from build123d import *

# Parameters (mm, degrees)
F0_W      = 20.75
F0_H      = 40.5
F2_DEPTH  = 2
F3_START  = 18
F1_W      = 20.75
F1_H      = 33.25
F3_DEPTH  = 2.25
F4_START  = -18
F4_DEPTH  = 2.25
F6_DEPTH  = 2.25
F8_DEPTH  = 2.25
F9_R      = 1.125
F10_DEPTH = 40.501
F11_R     = 1.27
F12_DEPTH = 2


with BuildPart() as f2:
    # F0 (on Top) → F2 (new body)
    with BuildSketch(Plane.XY):
        Rectangle(F0_W, F0_H)
    extrude(amount=F2_DEPTH)

    # F1 (on Front) → F3 (join)
    with BuildSketch(Plane.XZ.offset(F3_START)):
        with Locations((0, -16.625)):
            Rectangle(F1_W, F1_H)
    extrude(amount=F3_DEPTH)

    # F1 (on Front) → F4 (join)
    with BuildSketch(Plane.XZ.offset(F4_START)):
        with Locations((0, -16.625)):
            Rectangle(F1_W, F1_H)
    extrude(amount=-F4_DEPTH)

    # F5 (on face) → F6 (join, through all)
    with BuildSketch(Plane(origin=(0, 20.25, 0), x_dir=(-1, 0, 0), z_dir=(0, 1, 0))):
        Polygon((-10.375, -33.25), (-20.25, -33.25), (-20.25, -43.25), (20.25, -43.25), (20.25, -33.25), (10.375, -33.25), align=None)
    extrude(amount=-F6_DEPTH)

    # F7 (on face) → F8 (join, through all)
    with BuildSketch(Plane.XZ.offset(20.25)):
        Polygon((0, -33.25), (-20.25, -33.25), (-20.25, -43.25), (20.25, -43.25), (20.25, -33.25), align=None)
    extrude(amount=-F8_DEPTH)

    # F9 (on face) → F10 (cut, through all)
    with BuildSketch(Plane.XZ.offset(20.25)):
        with Locations((-13.25, -38.25)):
            Circle(F9_R)
        with Locations((13.25, -38.25)):
            Circle(F9_R)
    extrude(amount=-F10_DEPTH, mode=Mode.SUBTRACT)

    # F11 (on face) → F12 (cut, through all)
    with BuildSketch(Plane.XY.offset(2)):
        with BuildLine():
            ThreePointArc((-3.0697393815, 2.5959719896), (-3.3217599094, -8.4476517557), (6.286518813, -2.9973196771))
            ThreePointArc((6.286518813, -2.9973196771), (5.3868508916, 0.2609590453), (2.9427770074, 2.5959719896))
            ThreePointArc((2.9427770074, 2.5959719896), (-0.063481187, 0.0506803229), (-3.0697393815, 2.5959719896))
        make_face()
        with BuildLine():
            ThreePointArc((-3.0697393815, 2.5959719896), (-0.063481187, 3.3526803229), (2.9427770074, 2.5959719896))
            ThreePointArc((2.9427770074, 2.5959719896), (2.9740654362, 2.846461149), (2.984518813, 3.0986803229))
            ThreePointArc((2.984518813, 3.0986803229), (-0.315700361, 6.1362269461), (-3.0697393815, 2.5959719896))
        make_face()
        with BuildLine():
            ThreePointArc((-3.0697393815, 2.5959719896), (-0.063481187, 0.0506803229), (2.9427770074, 2.5959719896))
            ThreePointArc((2.9427770074, 2.5959719896), (-0.063481187, 3.3526803229), (-3.0697393815, 2.5959719896))
        make_face()
        with Locations((-0.063481187, -12.1413196771)):
            Circle(F11_R)
        with Locations((-0.063481187, 16.0526803229)):
            Circle(F11_R)
    extrude(amount=-F12_DEPTH, mode=Mode.SUBTRACT)


solid = f2.part
Read the model definition and answer for the solid it produces. Units are mm, in the model's axes. A direction names the side the tool comes from. Round coordinates to 2 decimals unless told otherwise and drop trailing zeros. Order: outer loops, then holes, each group sorted by start corner. A loop starts at its lowest first (then second) coordinate and runs counter-clockwise, first axis right, second up.
1) The part is cut by section D-D on y = 2. Write down the section's boundary in (x, z) (3 decimals), plus the area to 3 significant figures.
2) Straight lines are drawn through the part: L1, parallel to Y at x = 7, z = -1; L2, parallel to Y at x = 1, z = 0.5; L3, parallel to Z at x = -4.5, y = -14.5. For each, find the intervals that lie inside material, in ascending order.
3) The part is cut by section C-C on x = 13.25. Write down the section's boundary in (y, z) (3 decimals), plus the area to 3 significant figures.
4) The mould has two halves that part along X. Classify faces 1 (the face through (20.25, -19, -38)), 2 (the face through (0.619, 17.124, 1.014)), 3 (the face through (15, -19, -33.25)): released by +X, released by -X, zero draft, split by the parting line, or undercut.
5) For faces 4 (the face through (4, 4, 0)), 5 (the face through (-15, -19, -33.25)), 6 (the face through (15, 19, -33.25)), 7 (the face through (0, -19, -43.25)), determine the directions among +Z, -Z, +X, -X, +Y, -Y from which every point of the face is accessible in a straight line to the end or side of a thin tool.
6) Flat-ended cylindrical pins translate along their axes: pin 1 (2 mm diameter, centred on x = 13.25, z = -38.25, fed in from +Y); pin 2 (1.8 mm diameter, centred on x = 13, y = -19, fed in from +Z); pin 3 (10 mm diameter, centred on x = -0.06, y = 3.1, fed in from -Z). Find the tip coordinate at first contact, or state that the pin passes through.
7) The part is cut by section B-B on z = -31.5. Write down the section's boundary in (x, y) (3 decimals).
8) The part is cut by section A-A on z = -38.25. Write down the section's boundary in (x, y) (3 decimals), plus the area to 3 significant figures.
Resolved:
1. outline: (-10.375, 0) - (-3.981, 0) - (-3.981, 2) - (-10.375, 2) - close; (3.854, 0) - (10.375, 0) - (10.375, 2) - (3.854, 2) - close
1. area: 25.8 mm2
2. L1: y = -20.25 to -18, 18 to 20.25
2. L2: y = -20.25 to -12.84, -11.45 to -9.26, 5.96 to 15.36, 16.75 to 20.25
2. L3: z = 0 to 2
3. outline: (-20.25, -43.25) - (-18, -43.25) - (-18, -39.375) - (-20.25, -39.375) - close; (-20.25, -37.125) - (-18, -37.125) - (-18, -33.25) - (-20.25, -33.25) - close; (18, -43.25) - (20.25, -43.25) - (20.25, -39.375) - (18, -39.375) - close; (18, -37.125) - (20.25, -37.125) - (20.25, -33.25) - (18, -33.25) - close
3. area: 34.9 mm2
4. face 1: released by +X
4. face 2: undercut
4. face 3: zero draft
5. face 4: -Z, +X, -X
5. face 5: +Z, -X, +Y, -Y
5. face 6: +Z, +X, +Y, -Y
5. face 7: -Z, +X, -X, +Y, -Y
6. pin 1: passes through
6. pin 2: stops at z = -33.25
6. pin 3: stops at z = 0
7. outline: (-10.375, -20.25) - (10.375, -20.25) - (10.375, -18) - (-10.375, -18) - close; (-10.375, 18) - (10.375, 18) - (10.375, 20.25) - (-10.375, 20.25) - close
8. outline: (-20.25, -20.25) - (-14.375, -20.25) - (-14.375, -18) - (-20.25, -18) - close; (-20.25, 18) - (-14.375, 18) - (-14.375, 20.25) - (-20.25, 20.25) - close; (-12.125, -20.25) - (12.125, -20.25) - (12.125, -18) - (-12.125, -18) - close; (-12.125, 18) - (12.125, 18) - (12.125, 20.25) - (-12.125, 20.25) - close; (14.375, -20.25) - (20.25, -20.25) - (20.25, -18) - (14.375, -18) - close; (14.375, 18) - (20.25, 18) - (20.25, 20.25) - (14.375, 20.25) - close
8. area: 162 mm2
